Can you work these out from the model? Positions are in its coordinate system, mm. A direction names the side the tool comes from. Round coordinates to 2 decimals unless told otherwise and drop trailing zeros. Write each loop counter-clockwise with the first axis right and the second up, starting at its lowest first coordinate (ties: lowest second). Pieces come first, ordered by that corner, then holes. Notation, with made-up numbers: (60, 17.25) - (119, 17.25) arc R16 cw to (119, 39.25) - close; hole circle Ø1 at (77.5, 47). An arc over 180 degrees is marked (long way). One line per item, written item: value. Start each with the question number.
(1) I want a section at D-D on y = 15.5. List the corners of the cut face in (x, z) for me.
(2) If I drill on L1, parallel to Y at x = 36, z = 48; L2, parallel to Z at x = 51.5, y = 4.5; L3, parallel to Z at x = 38, y = 46, over which ranges is the centre line in solid material (lowest first)? Write a range as from..to.
(3) I want a section at A-A on x = 27.5. List the corners of the cut face in (y, z) for me, plus the area to 4 significant figures.
(4) On a 3-axis mill with a long thin cutter (end or side, diameter ignored), from which of +Z, -Z, +X, -X, +Y, -Y can I reach the whole of each face in a straight line? I mean faces 5 (the face through (11.21, 3.79, 22.28)), 6 (the face through (50, 19, 38)), 7 (the face through (35, 20, 45)), 8 (the face through (30, 35, 30)). Say none if no direction works.
(5) I'm going to push flat-ended pins straight in: pin 1 Ø8 at (y, z) = (9.5, 28.5) entering from -X; pin 2 Ø22 at (y, z) = (36, 42.5) entering from +X; pin 3 Ø9 at (x, y) = (38.5, 39) entering from +Z. Where does each tip first touch, or does it pass through?
(6) Thinking about a two-plate mould opening in Z: for faces 1 (the face through (39, 31, 40)), 2 (the face through (42, 25, 0)), 3 (the face through (7.69, 4.58, 26.04)), 4 (the face through (10, 10, 35)), which applies, +Z half, -Z half, draft (parallel to the pull), parting line (faces both ways), or undercut?
(7) I want a section at C-C on x = 4.5. List the corners of the cut face in (y, z) for me, plus the area to 3 significant figures.
from build123d import *

# Parameters (mm, degrees)
SKETCH1_W            = 70
SKETCH1_H            = 50
BOSS_EXTRUDE1_DEPTH  = 50
CUT_EXTRUDE1_DEPTH   = 50
SKETCH3_W            = 10
SKETCH3_H            = 30
CUT_EXTRUDE2_DEPTH   = 121
SKETCH4_W            = 20
SKETCH4_H            = 20
CUT_EXTRUDE3_DEPTH   = 121
CUT_EXTRUDE8_DEPTH   = 30
CUT_EXTRUDE9_DEPTH   = 0.0001
SKETCH11_W           = 20
SKETCH11_H           = 2
BOSS_EXTRUDE8_DEPTH  = 0.0001
SKETCH12_W           = 20
SKETCH12_H           = 20
CUT_EXTRUDE10_DEPTH  = 0.0001
CUT_EXTRUDE11_DEPTH  = 0.001
CUT_EXTRUDE12_DEPTH  = 0.001
CUT_EXTRUDE13_DEPTH  = 9.001
BOSS_EXTRUDE14_DEPTH = 0.0002
SKETCH18_W           = 30
SKETCH18_H           = 28.284271247
CUT_EXTRUDE17_DEPTH  = 23.0002
CUT_EXTRUDE18_DEPTH  = 0.0001


with BuildPart() as part:
    # Sketch1 → Boss-Extrude1 (new body)
    with BuildSketch(Plane.XY):
        with Locations((35, 25)):
            Rectangle(SKETCH1_W, SKETCH1_H)
    extrude(amount=BOSS_EXTRUDE1_DEPTH)

    # Sketch2 → Cut-Extrude1 (cut)
    with BuildSketch(Plane.XY.offset(50)):
        Polygon((0, 0), (20, 50), (0, 50), align=None)
    extrude(amount=-CUT_EXTRUDE1_DEPTH, mode=Mode.SUBTRACT)

    # Sketch3 → Cut-Extrude2 (cut)
    with BuildSketch(Plane(origin=(70, 0, 0), x_dir=(0, 0, -1), z_dir=(1, 0, 0))):
        with Locations((-45, 35)):
            Rectangle(SKETCH3_W, SKETCH3_H)
    extrude(amount=-CUT_EXTRUDE2_DEPTH, mode=Mode.SUBTRACT)

    # Sketch4 → Cut-Extrude3 (cut)
    with BuildSketch(Plane.XZ):
        with Locations((60, 40)):
            Rectangle(SKETCH4_W, SKETCH4_H)
    extrude(amount=-CUT_EXTRUDE3_DEPTH, mode=Mode.SUBTRACT)

    # Sketch5 → Cut-Extrude8 (cut)
    with BuildSketch(Plane.XY.offset(50)):
        Polygon((0, 0), (20, 20), (40, 50), (20, 50), align=None)
    extrude(amount=-CUT_EXTRUDE8_DEPTH, mode=Mode.SUBTRACT)

    # Sketch10 → Cut-Extrude9 (cut)
    with BuildSketch(Plane(origin=(0, 50, 0), x_dir=(1, 0, 0), z_dir=(0, 1, 0))):
        Polygon((20, 0), (50, 0), (50, -40), (40, -40), (40, -10), (20, -10), align=None)
    extrude(amount=-CUT_EXTRUDE9_DEPTH, mode=Mode.SUBTRACT)

    # Sketch11 → Boss-Extrude8 (add)
    with BuildSketch(Plane(origin=(0, 50, 0), x_dir=(1, 0, 0), z_dir=(0, 1, 0))):
        with Locations((60, -1)):
            Rectangle(SKETCH11_W, SKETCH11_H)
    extrude(amount=BOSS_EXTRUDE8_DEPTH)

    # Sketch12 → Cut-Extrude10 (cut)
    with BuildSketch(Plane(origin=(0, 50, 0), x_dir=(1, 0, 0), z_dir=(0, 1, 0))):
        with Locations((30, -20)):
            Rectangle(SKETCH12_W, SKETCH12_H)
    extrude(amount=-CUT_EXTRUDE10_DEPTH, mode=Mode.SUBTRACT)

    # Sketch14 → Cut-Extrude11 (cut)
    with BuildSketch(Plane(origin=(0, 0, 0), x_dir=(0, 0, 1), z_dir=(-0.707106781, 0.707106781, 0))):
        Polygon((20, 28.284271247), (50, 28.284271247), (50, 0), (30, 0), align=None)
    extrude(amount=-CUT_EXTRUDE11_DEPTH, mode=Mode.SUBTRACT)

    # Sketch15 → Cut-Extrude12 (cut)
    with BuildSketch(Plane(origin=(0, 0, 0), x_dir=(0, 0, 1), z_dir=(-0.928476691, 0.371390676, 0))):
        Polygon((0, 53.851648071), (30, 0), (0, 0), align=None)
    extrude(amount=-CUT_EXTRUDE12_DEPTH, mode=Mode.SUBTRACT)

    # Sketch16 → Cut-Extrude13 (cut)
    with BuildSketch(Plane(origin=(0.000928477, -0.000371391, 0), x_dir=(0, 0, 1), z_dir=(-0.928476691, 0.371390676, 0))):
        Polygon((20, 17.950549357), (29.998700133, 0.002333333), (20, 0.002333333), align=None)
    extrude(amount=-CUT_EXTRUDE13_DEPTH, mode=Mode.SUBTRACT)

    # Sketch17 → Boss-Extrude14 (add)
    with BuildSketch(Plane(origin=(0, 0, 0), x_dir=(0, 0, 1), z_dir=(-0.707106781, 0.707106781, 0))):
        Polygon((20, 28.284271247), (20, 19.529615861), (30, 0), align=None)
    extrude(amount=BOSS_EXTRUDE14_DEPTH)

    # Sketch18 → Cut-Extrude17 (cut)
    with BuildSketch(Plane(origin=(0.000707107, -0.000707107, 0), x_dir=(0, 0, 1), z_dir=(-0.707106781, 0.707106781, 0))):
        with Locations((35, 14.142135624)):
            Rectangle(SKETCH18_W, SKETCH18_H)
    extrude(amount=CUT_EXTRUDE17_DEPTH, mode=Mode.SUBTRACT)

    # Sketch19 → Cut-Extrude18 (cut)
    with BuildSketch(Plane(origin=(0, 0, 0), x_dir=(0, 0, 1), z_dir=(-0.928476691, 0.371390676, 0))):
        Polygon((17.214569927, 22.950549357), (20, 22.950549357), (20, 17.950549357), align=None)
    extrude(amount=-CUT_EXTRUDE18_DEPTH, mode=Mode.SUBTRACT)


solid = part.part
Established:
1. outline: (6.2, 0) - (70, 0) - (70, 30) - (50, 30) - (50, 50) - (15.5, 50) - (15.5, 20) - (6.2, 20) - close
2. L1: 0..20
2. L2: 0..30
2. L3: 0..40
3. outline: (0, 0) - (50, 0) - (50, 20) - (31.25, 20) - (31.25, 40) - (20, 40) - (20, 50) - (0, 50) - close
3. area: 1,825 mm2
4. face 5: -X
4. face 6: +Z, +X, +Y, -Y
4. face 7: +Z, +X, -X, +Y
4. face 8: +Z, -X, +Y
5. pin 1: x = 5.5
5. pin 2: x = 50
5. pin 3: z = 40
6. face 1: +Z half
6. face 2: -Z half
6. face 3: undercut
6. face 4: draft
7. outline: (0, 0) - (11.25, 0) - (11.25, 20) - (0, 20) - close; (0, 29.07) - (4.5, 26.74) - (4.5, 50) - (0, 50) - close
7. area: 324 mm2
